Source: CAD feature listing. Evaluate the final solid. Frame: model axes, mm. A direction names the side the tool comes from. Round coordinates to 2 decimals unless told otherwise and drop trailing zeros. Loops run counter-clockwise (first coordinate to the right, second up) from the corner with the lowest first, then second, coordinate; pieces in that order, holes last. Notation, with made-up numbers: M 0,6.5 L 43,6.5 A23 cw 43,14.5 Z; hole C 74,84.5 d10. An arc over 180 degrees is marked long. Answer as a JSON object with one key per item and string values.
Autodesk Inventor part; units mm, degrees
ref_plane "YZ Plane" through (0, 0, 0) normal (1, 0, 0) x (0, 1, 0)
ref_plane "XZ Plane" through (0, 0, 0) normal (0, 1, 0) x (-1, 0, 0)
ref_plane "XY Plane" through (0, 0, 0) normal (0, 0, 1) x (1, 0, 0)
sketch "Sketch1" plane through (0, 0, 0) normal (1, 0, 0) x (0, 1, 0)
  line L0 (0.0055, 3.1659) -> (2.7555, 1.5782)
  line L1 (2.7555, 1.5782) -> (2.7555, -1.5973)
  line L2 (2.7555, -1.5973) -> (0.0055, -3.185)
  line L3 (0.0055, -3.185) -> (-2.7445, -1.5973)
  line L4 (-2.7445, -1.5973) -> (-2.7445, 1.5782)
  line L5 (-2.7445, 1.5782) -> (0.0055, 3.1659)
  point P0 (0.0055, -0.0095)
  dimension "d1" = 5.5
extrude "Extrusion1" add sketch "Sketch1" along normal blind 11.182
sketch "Sketch2" plane through (0, 0, 0) normal (-1, 0, 0) x (0, 0, 1)
  circle A0 centre (0, 0) radius 1.5
  dimension "d4" = 3
extrude "Extrusion2" add sketch "Sketch2" along normal blind 7.619
sketch "Sketch3" plane through (11.182, 0, 0) normal (1, 0, 0) x (0, 0, -1)
  circle A0 centre (0, 0) radius 1.5
  dimension "d7" = 3
extrude "Extrusion3" cut sketch "Sketch3" against normal blind 6
properties part number "Spacer" material "Brass, Soft Yellow"
Item 1: Access query for faces 1 (the flat face through (-7.619, 0, 0)), 2 (the flat face through (0, -1.3, -1.4)), 3 (the cylindrical face through (8.22, 0.07, 1.5)). Directions: +Z, -Z, +X, -X, +Y, -Y. A direction counts if a zero-diameter tool reaches every point of the face in a straight line with its end or side. Return the directions, or none.
Answer sheet:
{"face 1": "+Z, -Z, -X, +Y, -Y", "face 2": "-X", "face 3": "+X"}
Item 2: Contact query for flat-ended pins moving along their axis: pin 1 Ø1 at (x, y) = (2, -2) entering from +Z; pin 2 Ø1.5 at (y, z) = (0, -0.5) entering from +X; pin 3 Ø3 at (x, z) = (6, 2) entering from +Y. Output: stop coordinate, or through.
Answer sheet:
{"pin 1": "stops at z = 2.3", "pin 2": "stops at x = 5.18", "pin 3": "stops at y = 2.76"}
Item 3: Section A-A on z = 0. Return the cut outline in (x, y), then the cut area to 3 significant figures.
Answer sheet:
{"outline": "M -7.62,-1.5 L 0,-1.5 L 0,-2.74 L 11.18,-2.74 L 11.18,-1.5 L 5.18,-1.5 L 5.18,1.5 L 11.18,1.5 L 11.18,2.76 L 0,2.76 L 0,1.5 L -7.62,1.5 Z", "area": "66.4 mm²"}
Item 4: Section D-D on x = 2.75. Return the cut outline in (y, z) (1 decimal).
Answer sheet:
{"outline": "M -2.7,-1.6 L 0,-3.2 L 2.8,-1.6 L 2.8,1.6 L 0,3.2 L -2.7,1.6 Z"}
Item 5: Pull-direction query (Z, two-part tool) for faces 4 (the flat face through (11.182, -1.3, -1.4)), 5 (the flat face through (5.513, 1.361, 2.383)), 6 (the flat face through (5.182, 0, 0)); classes: pulls with the +Z half, pulls with the -Z half, needs draft (parallel to the pull), parting line crosses it, or undercut.
Answer sheet:
{"face 4": "needs draft", "face 5": "pulls with the +Z half", "face 6": "undercut"}
Item 6: Section B-B on x = -3.25. Return the cut outline in (y, z), then the cut area to 3 significant figures.
Answer sheet:
{"outline": "C 0,0 d3", "area": "7.07 mm²"}
Item 7: Section C-C on y = 1.1. Return the cut outline in (x, z), then the cut area to 3 significant figures.
Answer sheet:
{"outline": "M -7.62,-1.02 L 0,-1.02 L 0,-2.55 L 11.18,-2.55 L 11.18,-1.02 L 5.18,-1.02 L 5.18,1.02 L 11.18,1.02 L 11.18,2.53 L 0,2.53 L 0,1.02 L -7.62,1.02 Z", "area": "60.2 mm²"}
Item 8: Line query: probe 1 along Y at (x, z) = (7.35, 0); probe 2 along X at (y, z) = (-2.45, -0.75); probe 3 along X at (y, z) = (0, 0.25). Output: solid intervals per line, ascending. Write a range as from..to.
Answer sheet:
{"probe 1": "y = -2.74..-1.5, 1.5..2.76", "probe 2": "x = 0..11.18", "probe 3": "x = -7.62..5.18"}
